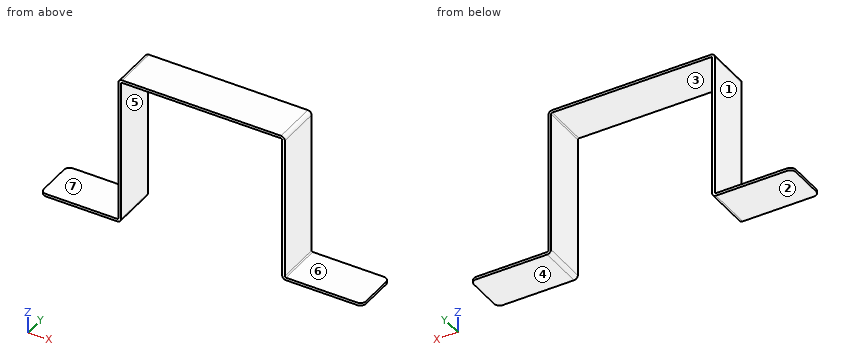
Autodesk Inventor part; units mm, degrees
ref_plane "YZ Plane" through (0, 0, 0) normal (1, 0, 0) x (0, 1, 0)
ref_plane "XZ Plane" through (0, 0, 0) normal (0, 1, 0) x (-1, 0, 0)
ref_plane "XY Plane" through (0, 0, 0) normal (0, 0, 1) x (1, 0, 0)
sketch "Sketch1" plane through (0, 0, 0) normal (0, 0, 1) x (1, 0, 0)
  line L0 (0, 0) -> (-184.15, 0)
  line L1 (-184.15, 0) -> (-184.15, 50.8)
  line L2 (-184.15, 50.8) -> (0, 50.8)
  line L3 (0, 50.8) -> (0, 0)
  dimension "d0" = 184.15
  dimension "d1" = 50.8
extrude "Plate1" add sketch "Sketch1" along normal blind 3.048
sketch "Sketch2" plane through (0, 0, 0) normal (1, 0, 0) x (0, 1, 0)
  line L0 (50.8, 0) -> (0, 0)
  line L1 (0, 0) -> (0, -165.1)
  line L2 (0, -165.1) -> (50.8, -165.1)
  line L3 (50.8, -165.1) -> (50.8, 0)
edge flange "Flange1" height 165.1 angle 90 thickness 3.048 bend radius 1.27 thickness toward (1, 0, 0) relief tear relief width 3.048 relief depth 1.524 corner gap 3.048 corner form 0 edges at (0, 25.4, 0) (-184.15, 25.4, 0) wall of the first edge with corners at (0, 50.8, 0) (0, 0, 0) (0, 0, -165.1) (0, 50.8, -165.1)
bend "Bend1"
corner "Corner1"
sketch "Sketch3" plane through (3.048, 50.8, -165.1) normal (0, 0, -1) x (-1, 0, 0)
  line L0 (0, -50.8) -> (0, 0)
  line L1 (0, 0) -> (-88.9, 0)
  line L2 (-88.9, 0) -> (-88.9, -50.8)
  line L3 (-88.9, -50.8) -> (0, -50.8)
edge flange "Flange2" height 88.9 angle 90 thickness 3.048 bend radius 1.27 thickness toward (0, 0, -1) relief tear relief width 3.048 relief depth 1.524 corner gap 3.048 corner form 0 edges at (3.048, 25.4, -165.1) (-187.198, 25.4, -165.1) wall of the first edge with corners at (3.048, 0, -165.1) (3.048, 50.8, -165.1) (91.948, 50.8, -165.1) (91.948, 0, -165.1)
bend "Bend2"
corner "Corner2"
fillet "Corner Round1" radius 6.35 4 edges at (-276.098, 0, -166.624) (-276.098, 50.8, -166.624) (91.948, 0, -166.624) (91.948, 50.8, -166.624)
equation "\"d3\" = BendReliefWidth"
equation "\"d4\" = BendReliefDepth"
equation "\"d5\" = MinimumRemnant"
equation "\"d6\" = BendRadius"
equation "\"d10\" = CornerReliefSize"
equation "\"d11\" = GapSize"
equation "\"d12\" = JacobiRadiusSize"
equation "\"d13\" = BendReliefWidth"
equation "\"d14\" = BendReliefDepth"
equation "\"d15\" = MinimumRemnant"
equation "\"d16\" = BendRadius"
equation "\"d20\" = CornerReliefSize"
equation "\"d21\" = GapSize"
equation "\"d22\" = JacobiRadiusSize"
equation "\"BendRadius\" = Thickness"
equation "\"BendReliefWidth\" = Thickness"
equation "\"BendReliefDepth\" = 0.5 * Thickness"
equation "\"CornerReliefSize\" = 4 * Thickness"
equation "\"MinimumRemnant\" = 2 * Thickness"
equation "\"TransitionRadius\" = BendRadius"
equation "\"JacobiRadiusSize\" = BendRadius"
equation "\"GapSize\" = Thickness"
equation "\"d2\" = BendRadius"
properties part number "battery staple"
Input: part model. Units: mm. Frame: model coordinates. Face numbers are marked on the shaded views. A direction names the side the tool comes from. Give positions to 0.01 mm unless a question says otherwise; leave off trailing zeros. Write each loop counter-clockwise with the first axis right and the second up, starting at its lowest first coordinate (ties: lowest second). Pieces come first, ordered by that corner, then holes. Notation, with made-up numbers: M 62.25,6 L 99.25,6 A15 cw 99.25,28 Z; hole C 66,-12.75 d7. An arc over 180 degrees is marked long. Write item = value, one per line. Start each with the question number.
1) Material intervals for line 1 along X through (y, z) = (3.5, -48); line 2 along Z through (x, y) = (-43, 46.5); line 3 along Z through (x, y) = (-198, 37.5), sorted ascending. Write a range as [from, to].
2) Cut plane A-A on z = -72.5. Return the cut outline in (x, y).
3) Cut plane C-C on x = 49. Return the cut outline in (y, z), then the cut area to 3 significant figures.
4) Draft query along X for the marked faces 1, 2 and 3. Return one class per face: +X half, -X half, draft (parallel to the pull), parting line (faces both ways), or undercut.
5) First-contact query: pin 1 Ø15 at (y, z) = (31.5, -75) entering from -X; pin 2 Ø3 at (y, z) = (42.5, -140) entering from +X; pin 3 Ø8 at (x, y) = (-147, 18) entering from -Z. Flat tips, straight axial feed; report the tip coordinate or a pass-through.
6) Reachability of the marked faces 4, 5, 6 and 7 from +Z, -Z, +X, -X, +Y, -Y: full face, straight path, thin tool, end or side. Return the list, or none.
7) Cut plane B-B on y = 10. Return the cut outline in (x, z).
Solved:
q1.line_1 = [-187.2, -184.15], [0, 3.05]
q1.line_2 = [0, 3.05]
q1.line_3 = [-168.15, -165.1]
q2.outline = M -187.2,0 L -184.15,0 L -184.15,50.8 L -187.2,50.8 Z; M 0,0 L 3.05,0 L 3.05,50.8 L 0,50.8 Z
q3.outline = M 0,-168.15 L 50.8,-168.15 L 50.8,-165.1 L 0,-165.1 Z
q3.area = 155 mm2
q4.face_1 = -X half
q4.face_2 = draft
q4.face_3 = undercut
q5.pin_1 = -187.2
q5.pin_2 = 3.05
q5.pin_3 = 0
q6.face_4 = -Z, +X, -X, +Y, -Y
q6.face_5 = -Z, +Y, -Y
q6.face_6 = +Z, +X, +Y, -Y
q6.face_7 = +Z, -X, +Y, -Y
q7.outline = M -276.1,-168.15 L -188.47,-168.15 A4.32 ccw -184.15,-163.83 L -184.15,-1.27 A1.27 cw -182.88,0 L -1.27,0 A1.27 cw 0,-1.27 L 0,-163.83 A4.32 ccw 4.32,-168.15 L 91.95,-168.15 L 91.95,-165.1 L 4.32,-165.1 A1.27 cw 3.05,-163.83 L 3.05,-1.27 A4.32 ccw -1.27,3.05 L -182.88,3.05 A4.32 ccw -187.2,-1.27 L -187.2,-163.83 A1.27 cw -188.47,-165.1 L -276.1,-165.1 Z
